Geometry check sheet. Reference: drawing and pictorial views, mm from the part's lowest x, y, z. Round coordinates to 2 decimals unless told otherwise and drop trailing zeros. Write each loop counter-clockwise with the first axis right and the second up, starting at its lowest first coordinate (ties: lowest second). Pieces come first, ordered by that corner, then holes. Notation, with made-up numbers: (89.5, 72) -> (145.5, 72) arc R36 cw to (145.5, 107) -> close; hole circle Ø1 at (-19.5, 23.25). An arc over 180 degrees is marked (long way). Answer as a JSON object with one key per item and string values. Group by question number.
(1) Draft check along X on the marked faces 1, 2 and 3. Enter one of: released by +X, released by -X, zero draft, split by the parting line, or undercut.
(2) Sectioned sample at C-C on x = 5. Record the cut outline in (y, z).
(3) Sectioned sample at A-A on z = 1. Record the cut outline in (x, y).
(4) Scan line: L1, parallel to Y at x = 4.5, z = 0.5. Record every from-to range of solid material in increasing order. Write a range as from..to.
(5) Sectioned sample at B-B on x = 6.04. Record the cut outline in (y, z).
(6) Sectioned sample at D-D on z = 1.75. Record the cut outline in (x, y), and give its area (3 significant figures).
(7) Gauge pin test, flat end, axial feed: pin 1 Ø0.6 at (x, z) = (3.5, 1) entering from -Y. Record the tip position at first contact, or that the pin passes through.
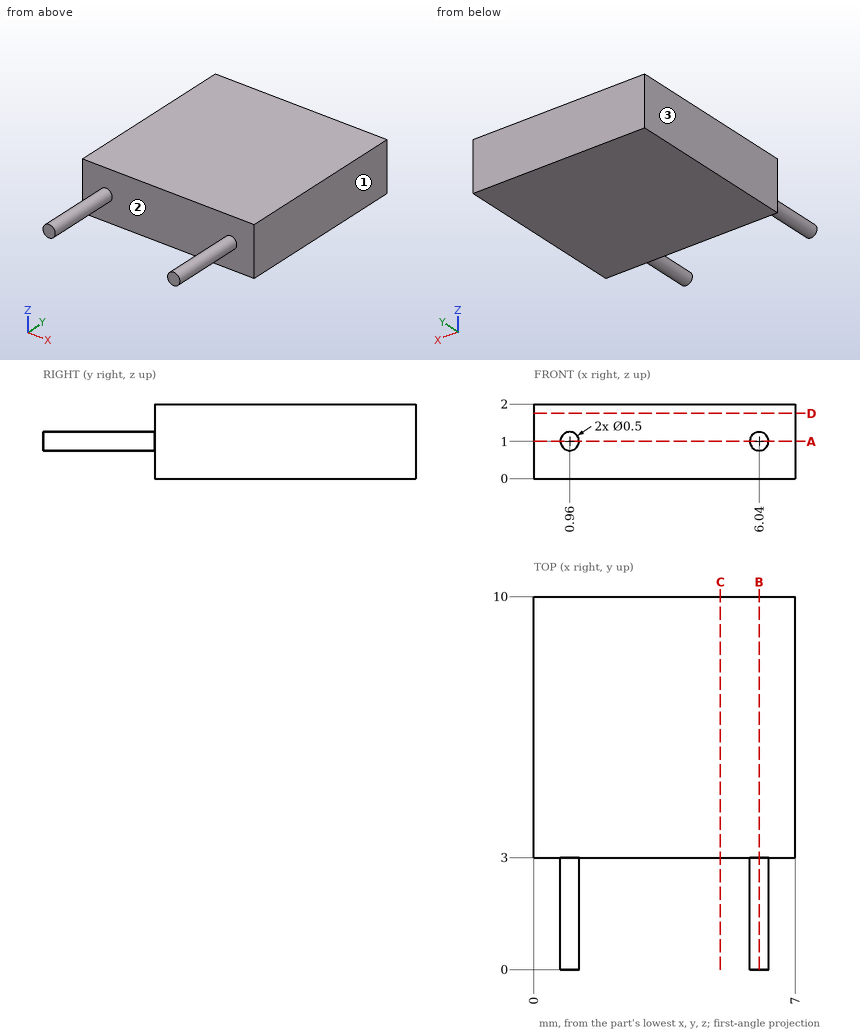
Computed values:
{
 "1": {"face 1": "released by +X", "face 2": "undercut", "face 3": "released by -X"},
 "2": {"outline": "(3, 0) -> (10, 0) -> (10, 2) -> (3, 2) -> close"},
 "3": {"outline": "(0, 3) -> (0.71, 3) -> (0.71, 0) -> (1.21, 0) -> (1.21, 3) -> (5.79, 3) -> (5.79, 0) -> (6.29, 0) -> (6.29, 3) -> (7, 3) -> (7, 10) -> (0, 10) -> close"},
 "4": {"L1": "3..10"},
 "5": {"outline": "(0, 0.75) -> (3, 0.75) -> (3, 0) -> (10, 0) -> (10, 2) -> (3, 2) -> (3, 1.25) -> (0, 1.25) -> close"},
 "6": {"outline": "(0, 3) -> (7, 3) -> (7, 10) -> (0, 10) -> close", "area": "49.0 mm2"},
 "7": {"pin 1": "y = 3"}
}
